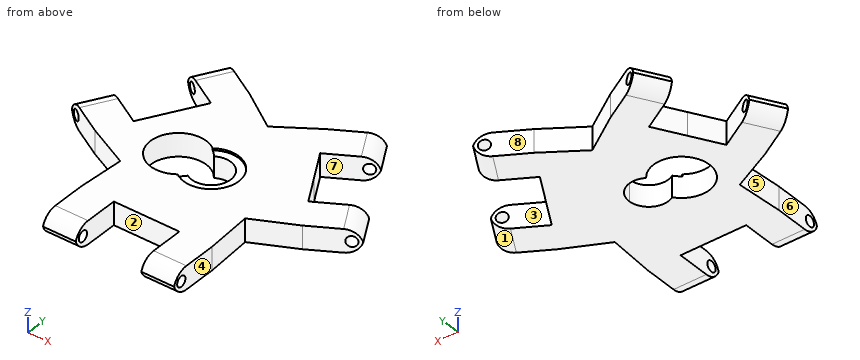
```python
from build123d import *

# Parameters (mm, degrees)
F0_W         = 10
F0_H         = 15
F1_DEPTH     = 7
F3_DEPTH     = 60
F4_R         = 1.6
F5_DEPTH     = 60
F6_R         = 1.6
F7_DEPTH     = 60
F8_T1_DEPTH  = 35
F8_T3_DEPTH  = 35
F8_T5_DEPTH  = 35
F8_T7_DEPTH  = 35
F8_T9_DEPTH  = 35
F8_T11_DEPTH = 35
F11_DEPTH    = 25
F12_R        = 8.4
F13_DEPTH    = 0.6


# Not quite as in the source:
# - a fillet or chamfer that OpenCascade refuses, or shapes differently, is made with other operations: its cross-section is extruded or revolved along the edge and cut away or added
# - a feature names something its author has since deleted; it is built from what else it names


with BuildPart() as f1:
    # F0 (on Top) → F1 (new body)
    with BuildSketch(Plane.XY):
        Polygon((-19.0935776077, -11.020506829), (-0.0410187244, -0.020506829), (-21.6916538191, 12.479493171), (-26.6916538191, 3.8192391331), (-31.6916538191, -4.8410149047), align=None)
        Polygon((-0.0410187244, 21.979493171), (-0.0410187244, -0.020506829), (21.6096163702, 12.479493171), (16.6096163702, 21.1397472088), (11.6096163702, 29.8000012467), align=None)
        Polygon((19.0115401588, -11.020506829), (-0.0410187244, -0.020506829), (-0.0410187244, -25.020506829), (9.9589812756, -25.020506829), (19.9589812756, -25.020506829), align=None)
        Polygon((-0.0410187244, -25.020506829), (-0.0410187244, -0.020506829), (-19.0935776077, -11.020506829), (-20.0410187244, -25.020506829), (-10.0410187244, -25.020506829), align=None)
        Polygon((-21.6916538191, 12.479493171), (-0.0410187244, -0.020506829), (-0.0410187244, 21.979493171), (-11.6916538191, 29.8000012467), (-16.6916538191, 21.1397472088), align=None)
        Polygon((21.6096163702, 12.479493171), (-0.0410187244, -0.020506829), (19.0115401588, -11.020506829), (31.6096163702, -4.8410149047), (26.6096163702, 3.8192391331), align=None)
        Polygon((-29.6820348758, 28.6397472088), (-16.6916538191, 21.1397472088), (-11.6916538191, 29.8000012467), (-24.6820348758, 37.3000012467), align=None)
        Polygon((-31.6916538191, -4.8410149047), (-26.6916538191, 3.8192391331), (-39.6820348758, 11.3192391331), (-44.6820348758, 2.6589850953), align=None)
        Polygon((39.5999974269, 11.3192391331), (26.6096163702, 3.8192391331), (31.6096163702, -4.8410149047), (44.5999974269, 2.6589850953), align=None)
        Polygon((11.6096163702, 29.8000012467), (16.6096163702, 21.1397472088), (29.5999974269, 28.6397472088), (24.5999974269, 37.3000012467), align=None)
        with Locations((-15.0410187244, -32.520506829)):
            Rectangle(F0_W, F0_H)
        with Locations((14.9589812756, -32.520506829)):
            Rectangle(F0_W, F0_H)
    extrude(amount=F1_DEPTH)

    # F2 (on face) → F3 (cut)
    with BuildSketch(Plane.YZ.offset(19.9589812756)):
        with BuildLine():
            ThreePointArc((-35.420506829, 3.5), (-37.020506829, 5.1), (-38.620506829, 3.5))
            ThreePointArc((-38.620506829, 3.5), (-37.020506829, 1.9), (-35.420506829, 3.5))
        make_face()
    extrude(amount=-F3_DEPTH, mode=Mode.SUBTRACT)

    # F4 (on face) → F5 (cut)
    with BuildSketch(Plane(origin=(9.9986250363, -17.3181265688, 0), x_dir=(0.8660254038, 0.5, 0), z_dir=(0.5, -0.8660254038, 0))):
        with Locations((36.9542233281, 3.5)):
            Circle(F4_R)
    extrude(amount=-F5_DEPTH, mode=Mode.SUBTRACT)

    # F6 (on face) → F7 (cut)
    with BuildSketch(Plane(origin=(9.9808656014, 17.2873663252, 0), x_dir=(-0.8660254038, 0.5, 0), z_dir=(0.5, 0.8660254038, 0))):
        with Locations((37.0252698429, 3.5)):
            Circle(F6_R)
    extrude(amount=-F7_DEPTH, mode=Mode.SUBTRACT)

    # F8: fillet of radius 5 on 12 edges, made by hand

    # F8_s2 → F8_t1 (cut)
    with BuildSketch(Plane.YZ.offset(-32.5410187244)):
        with BuildLine():
            ThreePointArc((-35.020506829, 7), (-38.556040735, 5.5355339059), (-40.020506829, 2))
            Line((-40.020506829, 2), (-40.020506829, 7))
            Line((-40.020506829, 7), (-35.020506829, 7))
        make_face()
        with BuildLine():
            ThreePointArc((-35.020506829, 0), (-38.556040735, 1.4644660941), (-40.020506829, 5))
            Line((-40.020506829, 5), (-40.020506829, 0))
            Line((-40.020506829, 0), (-35.020506829, 0))
        make_face()
    extrude(amount=F8_T1_DEPTH, mode=Mode.SUBTRACT)

    # F8_s4 → F8_t3 (cut)
    with BuildSketch(Plane.YZ.offset(-2.5410187244)):
        with BuildLine():
            ThreePointArc((-35.020506829, 0), (-38.556040735, 1.4644660941), (-40.020506829, 5))
            Line((-40.020506829, 5), (-40.020506829, 0))
            Line((-40.020506829, 0), (-35.020506829, 0))
        make_face()
        with BuildLine():
            ThreePointArc((-35.020506829, 7), (-38.556040735, 5.5355339059), (-40.020506829, 2))
            Line((-40.020506829, 2), (-40.020506829, 7))
            Line((-40.020506829, 7), (-35.020506829, 7))
        make_face()
    extrude(amount=F8_T3_DEPTH, mode=Mode.SUBTRACT)

    # F8_s6 → F8_t5 (cut)
    with BuildSketch(Plane(origin=(16.2486250363, -28.1434441161, 0), x_dir=(0, 0, 1), z_dir=(-0.5, 0.8660254038, 0))):
        with BuildLine():
            ThreePointArc((7, 34.9542233281), (5.5355339059, 38.489757234), (2, 39.9542233281))
            Line((2, 39.9542233281), (7, 39.9542233281))
            Line((7, 39.9542233281), (7, 34.9542233281))
        make_face()
        with BuildLine():
            ThreePointArc((0, 34.9542233281), (1.4644660941, 38.489757234), (5, 39.9542233281))
            Line((5, 39.9542233281), (0, 39.9542233281))
            Line((0, 39.9542233281), (0, 34.9542233281))
        make_face()
    extrude(amount=F8_T5_DEPTH, mode=Mode.SUBTRACT)

    # F8_s8 → F8_t7 (cut)
    with BuildSketch(Plane(origin=(1.2486250363, -2.1626820025, 0), x_dir=(0, 0, 1), z_dir=(-0.5, 0.8660254038, 0))):
        with BuildLine():
            ThreePointArc((7, 34.9542233281), (5.5355339059, 38.489757234), (2, 39.9542233281))
            Line((2, 39.9542233281), (7, 39.9542233281))
            Line((7, 39.9542233281), (7, 34.9542233281))
        make_face()
        with BuildLine():
            ThreePointArc((0, 34.9542233281), (1.4644660941, 38.489757234), (5, 39.9542233281))
            Line((5, 39.9542233281), (0, 39.9542233281))
            Line((0, 39.9542233281), (0, 34.9542233281))
        make_face()
    extrude(amount=F8_T7_DEPTH, mode=Mode.SUBTRACT)

    # F8_s10 → F8_t9 (cut)
    with BuildSketch(Plane(origin=(16.2308656014, 28.1126838725, 0), x_dir=(0, 0, 1), z_dir=(-0.5, -0.8660254038, 0))):
        with BuildLine():
            ThreePointArc((7, 35.0252698429), (5.5355339059, 38.5608037488), (2, 40.0252698429))
            Line((2, 40.0252698429), (7, 40.0252698429))
            Line((7, 40.0252698429), (7, 35.0252698429))
        make_face()
        with BuildLine():
            ThreePointArc((0, 35.0252698429), (1.4644660941, 38.5608037488), (5, 40.0252698429))
            Line((5, 40.0252698429), (0, 40.0252698429))
            Line((0, 40.0252698429), (0, 35.0252698429))
        make_face()
    extrude(amount=F8_T9_DEPTH, mode=Mode.SUBTRACT)

    # F8_s12 → F8_t11 (cut)
    with BuildSketch(Plane(origin=(1.2308656014, 2.131921759, 0), x_dir=(0, 0, 1), z_dir=(-0.5, -0.8660254038, 0))):
        with BuildLine():
            ThreePointArc((7, 35.0252698429), (5.5355339059, 38.5608037488), (2, 40.0252698429))
            Line((2, 40.0252698429), (7, 40.0252698429))
            Line((7, 40.0252698429), (7, 35.0252698429))
        make_face()
        with BuildLine():
            ThreePointArc((0, 35.0252698429), (1.4644660941, 38.5608037488), (5, 40.0252698429))
            Line((5, 40.0252698429), (0, 40.0252698429))
            Line((0, 40.0252698429), (0, 35.0252698429))
        make_face()
    extrude(amount=F8_T11_DEPTH, mode=Mode.SUBTRACT)

    # F10 (on face) → F11 (cut)
    with BuildSketch(Plane.XY.offset(7)):
        with BuildLine():
            ThreePointArc((-3.157625, -5.0430054887), (-1.9250328948, -2.6542242275), (-1.5, 0))
            Line((-1.5, 0), (-5.95, 0))
            ThreePointArc((-5.95, 0), (-5.2053034854, -2.8822414238), (-3.157625, -5.0430054887))
        make_face()
        with BuildLine():
            Line((-5.95, 0), (-1.5, 0))
            ThreePointArc((-1.5, 0), (-1.9250328948, 2.6542242275), (-3.157625, 5.0430054887))
            ThreePointArc((-3.157625, 5.0430054887), (-5.2053034854, 2.8822414238), (-5.95, 0))
        make_face()
        with BuildLine():
            ThreePointArc((-3.157625, 5.0430054887), (-1.9250328948, 2.6542242275), (-1.5, 0))
            ThreePointArc((-1.5, 0), (-1.9250328948, -2.6542242275), (-3.157625, -5.0430054887))
            ThreePointArc((-3.157625, -5.0430054887), (2.8822414238, -5.2053034854), (5.95, 0))
            ThreePointArc((5.95, 0), (2.8822414238, 5.2053034854), (-3.157625, 5.0430054887))
        make_face()
        with BuildLine():
            ThreePointArc((-3.157625, -5.0430054887), (-5.2053034854, -2.8822414238), (-5.95, 0))
            ThreePointArc((-5.95, 0), (-5.2053034854, 2.8822414238), (-3.157625, 5.0430054887))
            ThreePointArc((-3.157625, 5.0430054887), (-18.5, 0), (-3.157625, -5.0430054887))
        make_face()
    extrude(amount=-F11_DEPTH, mode=Mode.SUBTRACT)

    # F12 (on face) → F13 (cut)
    with BuildSketch(Plane.XY.offset(7)):
        Circle(F12_R)
    extrude(amount=-F13_DEPTH, mode=Mode.SUBTRACT)


solid = f1.part
```
Can you work these out from the model? Positions are in its coordinate system, mm. Face numbers are marked on the shaded views. A direction names the side the tool comes from. Round coordinates to 2 decimals unless told otherwise and drop trailing zeros. Order: outer loops, then holes, each group sorted by start corner. A loop starts at its lowest first (then second) coordinate and runs counter-clockwise, first axis right, second up.
(1) If I drill on L1, parallel to X at y = -31, z = 5; L2, parallel to X at y = -3, z = 5; L3, parallel to Y at x = 12.75, z = 3.5, over which ranges is the centre line in solid material (lowest first)?
Results are:
L1: x = -20.04 to -10.04, 9.96 to 19.96
L2: x = -34.88 to -17.95, 5.14 to 34.8
L3: y = -39.79 to -38.62, -35.42 to 30.46
(2) If we section it at B-B (x = -8.5): Please give me the cut outline in (y, z), plus the area to 3 significant figures.
Results are:
outline: (-25.02, 0) - (-8.37, 0) - (-8.37, 7) - (-25.02, 7) - close; (8.37, 0) - (27.66, 0) - (27.66, 7) - (8.37, 7) - close
area: 252 mm2
(3) If we section it at A-A (y = -29): Please give me the cut outline in (x, z), plus the area to 3 significant figures.
Results are:
outline: (-20.04, 0) - (-10.04, 0) - (-10.04, 7) - (-20.04, 7) - close; (9.96, 0) - (19.96, 0) - (19.96, 7) - (9.96, 7) - close
area: 140 mm2
(4) We'd pull the mould along X, two halves only. Please class the marked faces 6, 7 and 8: +X half, -X half, draft (parallel to the pull), parting line (faces both ways), or undercut.
Results are:
face 6: -X half
face 7: +X half
face 8: undercut
(5) I'm going to push flat-ended pins straight in: pin 1 (6 mm diameter, centred on x = 25, y = -28.5, fed in from -Z); pin 2 (1.5 mm diameter, centred on x = -8.5, z = 4.5, fed in from -Y); pin 3 (3 mm diameter, centred on x = 18, z = 5.5, fed in from -Y); pin 4 (4 mm diameter, centred on y = 0, z = 2, fed in from +X). Where does each tip first touch, or does it pass through?
Results are:
pin 1: passes through
pin 2: stops at y = -25.02
pin 3: stops at y = -39.6
pin 4: stops at x = 43.46
(6) On a 3-axis mill with a long thin cutter (end or side, diameter ignored), from which of +Z, -Z, +X, -X, +Y, -Y can I reach the whole of each face in a straight line? I mean the marked faces 1, 2, 3, 4 and 5. Say none if no direction works.
Results are:
face 1: -Z, +X, +Y
face 2: +Z, -Z, -Y
face 3: +Z, -Z
face 4: +Z, -Z, +X, -Y
face 5: +Z, -Z, -X
(7) If we section it at D-D (y = -20): Please give me the cut outline in (x, z).
Results are:
outline: (-19.7, 0) - (19.62, 0) - (19.62, 7) - (-19.7, 7) - close
(8) If we section it at C-C (x = 2): Please give me the cut outline in (y, z).
Results are:
outline: (-25.02, 0) - (-5.6, 0) - (-5.6, 6.4) - (-8.16, 6.4) - (-8.16, 7) - (-25.02, 7) - close; (5.6, 0) - (23.35, 0) - (23.35, 7) - (8.16, 7) - (8.16, 6.4) - (5.6, 6.4) - close
